Check sheet for the drawn part. Datum: minimum x, y, z corner. Units: mm. A direction names the side the tool comes from. Coordinates: 2 decimals unless noted, no trailing zeros. Write each loop counter-clockwise with the first axis right and the second up, starting at its lowest first coordinate (ties: lowest second). Pieces come first, ordered by that corner, then holes. Notation, with made-up numbers: (50.5, 83.5) - (83.5, 83.5) arc R14 ccw to (83.5, 108.5) - close; hole circle Ø10 at (55, 49). An arc over 180 degrees is marked (long way). Use one line per item in the form item = value. Start each with the question number.
1. Cross-section at B-B on y = 103.5. Record the boundary of the cut face in (x, z).
2. Draft check along X on the marked faces 3, 4 and 5. Enter one of: +X half, -X half, draft (parallel to the pull), parting line (faces both ways), or undercut.
3. Cross-section at D-D on y = 15. Record the boundary of the cut face in (x, z).
4. Cross-section at C-C on x = 13.5. Record the boundary of the cut face in (y, z), then the cut area to 3 significant figures.
5. Go/stop test with a flat-tipped pin: pin 1 Ø12 at (x, z) = (7.5, 4) entering from -Y. Record where the tip stops, or that it passes through.
6. Scan lines: line 1 along X through (y, z) = (168.5, 15); line 2 along Z through (x, y) = (1.5, 214.5). Record each from-to range of solid material in increasing order.
7. Tool access check on the marked faces 1 and 2. Record the directions out of +Z, -Z, +X, -X, +Y, -Y that give a thin tool (end or side, any length) a straight path to the whole face; none if there is none.
8. Cross-section at A-A on z = 12.5. Give the number of separate pieces and of enclosed holes in the cut face, then the cut area to 3 significant figures.
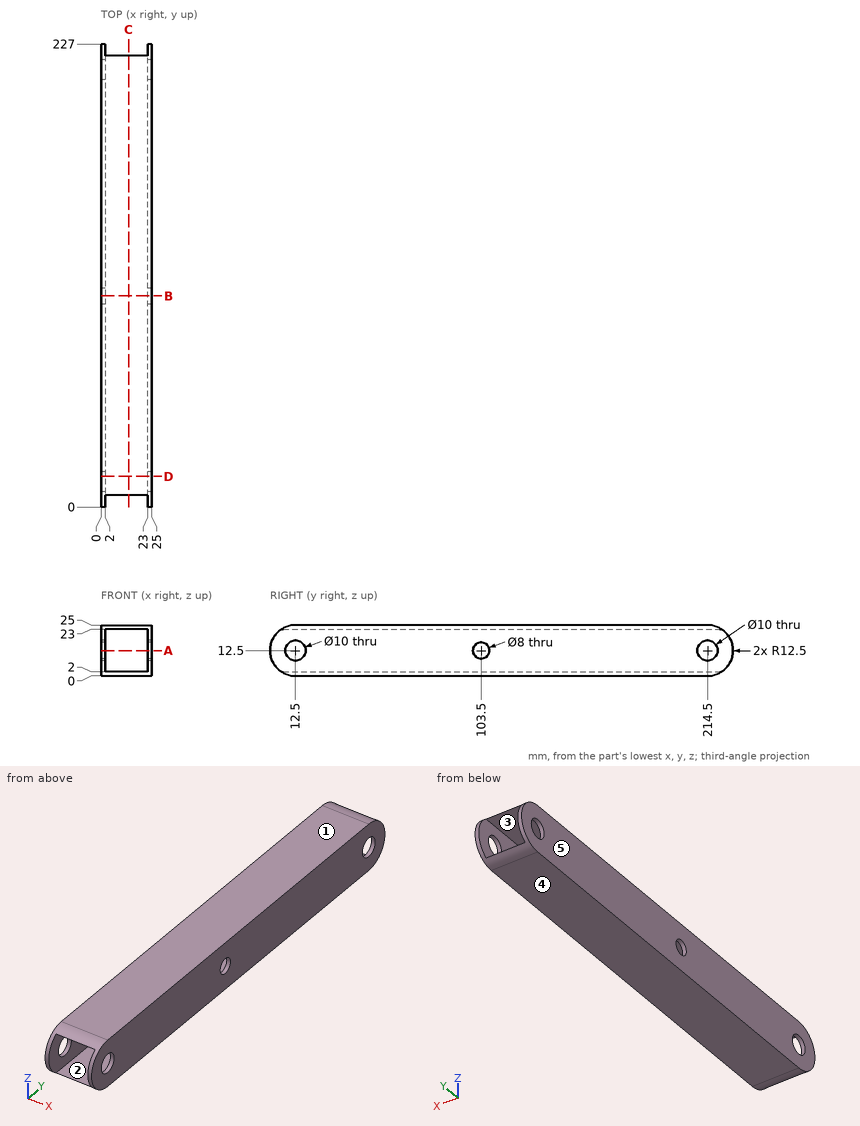
Final values:
q1.outline = (0, 0) - (25, 0) - (25, 8.5) - (23, 8.5) - (23, 2) - (2, 2) - (2, 8.5) - (0, 8.5) - close; (0, 16.5) - (2, 16.5) - (2, 23) - (23, 23) - (23, 16.5) - (25, 16.5) - (25, 25) - (0, 25) - close
q2.face_3 = undercut
q2.face_4 = draft
q2.face_5 = -X half
q3.outline = (0, 0) - (25, 0) - (25, 8.17) - (23, 8.17) - (23, 2) - (2, 2) - (2, 8.17) - (0, 8.17) - close; (0, 16.83) - (2, 16.83) - (2, 23) - (23, 23) - (23, 16.83) - (25, 16.83) - (25, 25) - (0, 25) - close
q4.outline = (5.72, 2) arc R12.5 ccw to (12.5, 0) - (214.5, 0) arc R12.5 ccw to (221.28, 2) - close; (5.72, 23) - (221.28, 23) arc R12.5 ccw to (214.5, 25) - (12.5, 25) arc R12.5 ccw to start
q4.area = 845 mm²
q5.pin_1 = 1.59
q6.line_1 = 0 to 2, 23 to 25
q6.line_2 = 0 to 7.5, 17.5 to 25
q7.face_1 = +Z, +X, -X, +Y, -Y
q7.face_2 = +Y, -Y
q8.separate_pieces = 8
q8.enclosed_holes = 0
q8.area = 796 mm²
